from build123d import *

# Parameters (mm, degrees)
CROQUIS1_R              = 16.9
CROQUIS1_R_2            = 13.9
SALIENTE_EXTRUIR1_DEPTH = 37.9
CROQUIS2_R              = 6.3
CORTAR_EXTRUIR1_DEPTH   = 20.8
CHAFL_N1_SIZE           = 3


with BuildPart() as part:
    # Croquis1 → Saliente-Extruir1 (new, symmetric)
    with BuildSketch(Plane.XY):
        Circle(CROQUIS1_R)
        Circle(CROQUIS1_R_2, mode=Mode.SUBTRACT)
    extrude(amount=SALIENTE_EXTRUIR1_DEPTH, both=True)

    # Croquis2 → Cortar-Extruir1 (cut)
    with BuildSketch(Plane(origin=(0, 16.9, 0), x_dir=(1, 0, 0), z_dir=(0, 1, 0))):
        with Locations(Location((0, 0, 0), (0, 0, 270))):
            Circle(CROQUIS2_R)
    extrude(amount=-CORTAR_EXTRUIR1_DEPTH, mode=Mode.SUBTRACT)

    # Chaflán1
    chafl_n1_edges = [part.edges().sort_by_distance(p)[0] for p in [
        (-13.9, 0, -37.9),
        (-13.9, 0, 37.9),
    ]]
    chamfer(chafl_n1_edges, length=CHAFL_N1_SIZE - 0.0001)  # a hair under: the kernel refuses the full size


solid = part.part
Build history of the part. All positions in model axes, mm. A direction names the side the tool comes from. Round coordinates to 2 decimals unless told otherwise and drop trailing zeros. Write each loop counter-clockwise with the first axis right and the second up, starting at its lowest first coordinate (ties: lowest second). Pieces come first, ordered by that corner, then holes. Notation, with made-up numbers: M -28,56.5 L 22,56.5 A12 cw 22,74.5 Z; hole C 64.5,-26.5 d1. An arc over 180 degrees is marked long. Answer in a Markdown table with one row per item.
1. Saw through at B-B (x = 0). State how many separate pieces and enclosed holes the cut face has, and give its area (3 significant figures).
Geometry check:
| item | result |
|---|---|
| separate pieces | 3 |
| enclosed holes | 0 |
| area | 399 mm2 |
2. Flat gauge pins, fed straight in: P1, Ø2, axis at x = -6.5, z = 17, coming from the -Y side; P2, Ø5, axis at y = -12, z = 25, coming from the +X side; P3, Ø10, axis at x = 9, z = 16.5, coming from the +Y side. Where does each tip first touch, or does it go through?
Geometry check:
| item | result |
|---|---|
| P1 | y = -15.98 |
| P2 | x = 13.98 |
| P3 | y = 16.42 |
3. Which spindle directions (+Z, -Z, +X, -X, +Y, -Y) get a long thin tool onto all of the face, cutting with end or side? Do faces 3 (the face through (0.277, 14.677, -6.294)), 4 (the face through (-3.01, -13.57, -0.49)). Say none if no direction does.
Geometry check:
| item | result |
|---|---|
| face 3 | +Y |
| face 4 | +Z, -Z |
4. Saw through at D-D (z = 0). List the corners of the cut face in (x, y).
Geometry check:
| item | result |
|---|---|
| outline | M -6.3,12.39 L -6.3,15.68 A16.9 ccw long 6.3,15.68 L 6.3,12.39 A13.9 cw long Z |
5. Saw through at C-C (z = -28). List the corners of the cut face in (x, y), and give its area (3 significant figures).
Geometry check:
| item | result |
|---|---|
| outline | C 0,0 d33.8; hole C 0,0 d27.8 |
| area | 290 mm2 |
6. Probe L1, parallel to X at y = -4.5, z = -30; L2, parallel to Y at x = -5, z = -27.5; L3, parallel to X at y = 2, z = -31.5. List the from-to ranges inside material, lowest first. Write a range as [from, to].
Geometry check:
| item | result |
|---|---|
| L1 | [-16.29, -13.15], [13.15, 16.29] |
| L2 | [-16.14, -12.97], [12.97, 16.14] |
| L3 | [-16.78, -13.76], [13.76, 16.78] |
7. Mould opens along X. For faces 1 (the face through (-3.054, -13.753, 35.088)), 2 (the face through (7.798, -14.993, 0.531)) say: +X half, -X half, draft (parallel to the pull), parting line (faces both ways), or undercut.
Geometry check:
| item | result |
|---|---|
| face 1 | undercut |
| face 2 | parting line |
